from build123d import *

# Parameters (mm, degrees)
EXTRUDE_1_DEPTH     = 3
SKETCH_3_R          = 1.6
CUT_EXTRUDE_1_DEPTH = 3


with BuildPart() as part:
    # 草图1 → 凸台-拉伸1 (new body)
    with BuildSketch(Plane.XY):
        Polygon((0, 0), (0, 20), (60, 20), (60, 0), (40, -20), (40, -25), (20, -25), (20, -20), align=None)
    extrude(amount=EXTRUDE_1_DEPTH)

    # 草图3 → 切除-拉伸1 (cut)
    with BuildSketch(Plane.XY.offset(3)):
        with Locations((26, -5)):
            Circle(SKETCH_3_R)
        with Locations((34, -5)):
            Circle(SKETCH_3_R)
        with Locations((26, -20)):
            Circle(SKETCH_3_R)
        with Locations((34, -20)):
            Circle(SKETCH_3_R)
        with Locations((26, -12.5)):
            Circle(SKETCH_3_R)
        with Locations((34, -12.5)):
            Circle(SKETCH_3_R)
        with Locations((5, 14)):
            Circle(SKETCH_3_R)
        with Locations((5, 6)):
            Circle(SKETCH_3_R)
        with Locations((14, 14)):
            Circle(SKETCH_3_R)
        with Locations((14, 6)):
            Circle(SKETCH_3_R)
        with Locations((55, 14)):
            Circle(SKETCH_3_R)
        with Locations((55, 6)):
            Circle(SKETCH_3_R)
        with Locations((46, 14)):
            Circle(SKETCH_3_R)
        with Locations((46, 6)):
            Circle(SKETCH_3_R)
    extrude(amount=-CUT_EXTRUDE_1_DEPTH, mode=Mode.SUBTRACT)


solid = part.part
Could you check a few things on this model? Use its own coordinates, in mm. A direction names the side the tool comes from. Coordinates: 2 decimals unless noted, no trailing zeros. Order: outer loops, then holes, each group sorted by start corner. A loop starts at its lowest first (then second) coordinate and runs counter-clockwise, first axis right, second up. Notation, with made-up numbers: (-2, 9.25) - (33, 9.25) arc R20 cw to (33, 14.25) - close; hole circle Ø4 at (18, -12.75). An arc over 180 degrees is marked (long way). Answer in a Markdown table with one row per item. Add a question column.
(1) If we section it at B-B, the plane y = -5: Please give me the cut outline in (x, z).
(2) On a 3-axis mill with a long thin cutter (end or side, diameter ignored), from which of +Z, -Z, +X, -X, +Y, -Y can I reach the whole of each face in a straight line? I mean faces 1 (the face through (32.82, -18.92, 1.52)), 2 (the face through (40, -22, 1)), 3 (the face through (20, -23, 1)). Say none if no direction works.
(3) If we section it at A-A, the plane x = 55: Please give me the cut outline in (y, z), then the cut area to 3 significant figures.
(4) If we section it at C-C, the plane y = 14: Please give me the cut outline in (x, z), then the cut area to 3 significant figures.
(5) If we section it at D-D, the plane z = 2.05: State how many separate pieces and enclosed holes the cut face has, then the cut area to 3 significant figures.
(6) I need wall thicknesses on L1, parallel to X at y = -21, z = 0.55; L2, parallel to Y at x = 5, z = 2.25; L3, parallel to Y at x = 34, z = 1.5. Which ranges of each line are inside material? Lowest first, please.
(7) Will these pins go through, and if not, where does the flat tip stop? pin 1 (1.5 mm diameter, centred on x = 42.5, y = -20, fed in from -Z); pin 2 (1.5 mm diameter, centred on y = -23.5, z = 2, fed in from -X); pin 3 (0.9 mm diameter, centred on y = -21.5, z = 1, fed in from +X).
(8) If we mould it in two halves opening along X, with no side actions, what happens to faces 4 (the face through (10, -10, 1)), 5 (the face through (45.65, 4.44, 1.52)), 6 (the face through (30, 3, 0)), 7 (the face through (4.65, 4.44, 1.52))? For each: released by +X, released by -X, zero draft, split by the parting line, or undercut.
Results are:
| question | item | result |
|---|---|---|
| 1 | outline | (5, 0) - (24.4, 0) - (24.4, 3) - (5, 3) - close; (27.6, 0) - (32.4, 0) - (32.4, 3) - (27.6, 3) - close; (35.6, 0) - (55, 0) - (55, 3) - (35.6, 3) - close |
| 2 | face 1 | +Z, -Z |
| 2 | face 2 | +Z, -Z, +X, -Y |
| 2 | face 3 | +Z, -Z, -X, -Y |
| 3 | outline | (-5, 0) - (4.4, 0) - (4.4, 3) - (-5, 3) - close; (7.6, 0) - (12.4, 0) - (12.4, 3) - (7.6, 3) - close; (15.6, 0) - (20, 0) - (20, 3) - (15.6, 3) - close |
| 3 | area | 55.8 mm2 |
| 4 | outline | (0, 0) - (3.4, 0) - (3.4, 3) - (0, 3) - close; (6.6, 0) - (12.4, 0) - (12.4, 3) - (6.6, 3) - close; (15.6, 0) - (44.4, 0) - (44.4, 3) - (15.6, 3) - close; (47.6, 0) - (53.4, 0) - (53.4, 3) - (47.6, 3) - close; (56.6, 0) - (60, 0) - (60, 3) - (56.6, 3) - close |
| 4 | area | 142 mm2 |
| 5 | separate pieces | 1 |
| 5 | enclosed holes | 14 |
| 5 | area | 1,990 mm2 |
| 6 | L1 | x = 20 to 24.75, 27.25 to 32.75, 35.25 to 40 |
| 6 | L2 | y = -5 to 4.4, 7.6 to 12.4, 15.6 to 20 |
| 6 | L3 | y = -25 to -21.6, -18.4 to -14.1, -10.9 to -6.6, -3.4 to 20 |
| 7 | pin 1 | passes through |
| 7 | pin 2 | stops at x = 20 |
| 7 | pin 3 | stops at x = 40 |
| 8 | face 4 | released by -X |
| 8 | face 5 | undercut |
| 8 | face 6 | zero draft |
| 8 | face 7 | undercut |
